from build123d import *

# Parameters (mm, degrees)
BOSS_EXTRUDE1_DEPTH = 5.4
SKETCH3_W           = 0.6
SKETCH3_H           = 0.5
BOSS_EXTRUDE3_DEPTH = 4.7
SKETCH4_W           = 2
SKETCH4_H           = 2
BOSS_EXTRUDE4_DEPTH = 2
SKETCH5_W           = 1.2
SKETCH5_H           = 2.4
CUT_EXTRUDE1_DEPTH  = 4.6


with BuildPart() as part:
    # Sketch1 → Boss-Extrude1 (new body)
    with BuildSketch(Plane(origin=(0, 0, 0), x_dir=(1, 0, 0), z_dir=(0, 1, 0))):
        with BuildLine():
            Line((-5.8, -2), (-0.3, -2))
            ThreePointArc((-0.3, -2), (0, -1.7), (0.3, -2))
            Line((0.3, -2), (5.8, -2))
            Line((5.8, -2), (5.8, 2))
            Line((5.8, 2), (0.3, 2))
            ThreePointArc((0.3, 2), (0, 1.7), (-0.3, 2))
            Line((-0.3, 2), (-5.8, 2))
            Line((-5.8, 2), (-5.8, -2))
        make_face()
    extrude(amount=BOSS_EXTRUDE1_DEPTH)

    # Sketch3 → Boss-Extrude3 (add)
    with BuildSketch(Plane.XZ):
        Rectangle(SKETCH3_W, SKETCH3_H)
        with Locations((2.5, 0)):
            Rectangle(SKETCH3_W, SKETCH3_H)
        with Locations((-2.5, 0)):
            Rectangle(SKETCH3_W, SKETCH3_H)
    extrude(amount=BOSS_EXTRUDE3_DEPTH)

    # Sketch4 → Boss-Extrude4 (add)
    with BuildSketch(Plane(origin=(0, 5.4, 0), x_dir=(1, 0, 0), z_dir=(0, 1, 0))):
        with Locations((-1.3, 0)):
            Rectangle(SKETCH4_W, SKETCH4_H)
    extrude(amount=BOSS_EXTRUDE4_DEPTH)

    # Sketch5 → Cut-Extrude1 (cut)
    with BuildSketch(Plane(origin=(0, 5.4, 0), x_dir=(1, 0, 0), z_dir=(0, 1, 0))):
        with Locations((5.8, 0)):
            Rectangle(SKETCH5_W, SKETCH5_H)
    cut_extrude1 = extrude(amount=-CUT_EXTRUDE1_DEPTH, mode=Mode.SUBTRACT)

    # Mirror1: Cut-Extrude1 across plane
    add(cut_extrude1.mirror(Plane(origin=(0, 0, 0), x_dir=(0, 0, 1), z_dir=(1, 0, 0))), mode=Mode.SUBTRACT)


solid = part.part
Geometry: final body of the model. Coordinates: model frame, mm. A direction names the side the tool comes from. Give positions to 0.01 mm unless a question says otherwise; leave off trailing zeros. Write each loop counter-clockwise with the first axis right and the second up, starting at its lowest first coordinate (ties: lowest second). Pieces come first, ordered by that corner, then holes. Notation, with made-up numbers: (11, 31.25) -> (47, 31.25) arc R20 ccw to (47, 62.25) -> close; hole circle Ø2 at (40, -34). An arc over 180 degrees is marked (long way). Answer as a JSON object with one key per item and string values.
1. Cut plane B-B on x = 2.5. Output: boundary loops of the cut face in (y, z).
Ans:
{"outline": "(-4.7, -0.25) -> (0, -0.25) -> (0, -2) -> (5.4, -2) -> (5.4, 2) -> (0, 2) -> (0, 0.25) -> (-4.7, 0.25) -> close"}
2. Cut plane D-D on z = -0.75. Output: boundary loops of the cut face in (x, y).
Ans:
{"outline": "(-5.8, 0) -> (5.8, 0) -> (5.8, 0.8) -> (5.2, 0.8) -> (5.2, 5.4) -> (-0.3, 5.4) -> (-0.3, 7.4) -> (-2.3, 7.4) -> (-2.3, 5.4) -> (-5.2, 5.4) -> (-5.2, 0.8) -> (-5.8, 0.8) -> close"}
3. Access query for faces 5 (the flat face through (-1, 6, -1)), 6 (the flat face through (-0.3, 6, 0)), 7 (the flat face through (-1, 6, 1)), 8 (the flat face through (3, 3, -2)). Directions: +Z, -Z, +X, -X, +Y, -Y. A direction counts if a zero-diameter tool reaches every point of the face in a straight line with its end or side. Return the directions, or none.
Ans:
{"face 5": "-Z, +X, -X, +Y", "face 6": "+Z, -Z, +X, +Y", "face 7": "+Z, +X, -X, +Y", "face 8": "-Z, +X, -X, +Y, -Y"}
4. Ray query, probe 1 along X at (y, z) = (-4, 0.2); probe 2 along Y at (x, z) = (0.75, 0.6); probe 3 along X at (y, z) = (2.5, -0.1). Return the intervals inside material, ascending. Write a range as from..to.
Ans:
{"probe 1": "x = -2.8..-2.2, -0.3..0.3, 2.2..2.8", "probe 2": "y = 0..5.4", "probe 3": "x = -5.2..5.2"}
5. Cut plane C-C on y = 2.5. Output: boundary loops of the cut face in (x, z).
Ans:
{"outline": "(-5.8, -2) -> (-0.3, -2) arc R0.3 cw to (0.3, -2) -> (5.8, -2) -> (5.8, -1.2) -> (5.2, -1.2) -> (5.2, 1.2) -> (5.8, 1.2) -> (5.8, 2) -> (0.3, 2) arc R0.3 cw to (-0.3, 2) -> (-5.8, 2) -> (-5.8, 1.2) -> (-5.2, 1.2) -> (-5.2, -1.2) -> (-5.8, -1.2) -> close"}
6. Cut plane A-A on y = -3. Output: boundary loops of the cut face in (x, z), and give its area (3 significant figures).
Ans:
{"outline": "(-2.8, -0.25) -> (-2.2, -0.25) -> (-2.2, 0.25) -> (-2.8, 0.25) -> close; (-0.3, -0.25) -> (0.3, -0.25) -> (0.3, 0.25) -> (-0.3, 0.25) -> close; (2.2, -0.25) -> (2.8, -0.25) -> (2.8, 0.25) -> (2.2, 0.25) -> close", "area": "0.900 mm^2"}
7. Contact query for flat-ended pins moving along their axis: pin 1 (1.6 mm diameter, centred on y = 7, z = 0, fed in from -X); pin 2 (1 mm diameter, centred on x = 3, z = 0, fed in from +Y); pin 3 (2 mm diameter, centred on x = 1.5, y = -2.5, fed in from +Z). Output: stop coordinate, or through.
Ans:
{"pin 1": "stops at x = -2.3", "pin 2": "stops at y = 5.4", "pin 3": "stops at z = 0.25"}
8. Mould query, pull axis Z, two halves, no side actions, for faces 1 (the flat face through (5.2, 3, 0)), 2 (the flat face through (-2.3, 6, 0)), 3 (the flat face through (-3, 3, 2)), 4 (the flat face through (-5.2, 3, 0)). Classes: pulls with the +Z half, pulls with the -Z half, needs draft (parallel to the pull), parting line crosses it, or undercut.
Ans:
{"face 1": "undercut", "face 2": "needs draft", "face 3": "pulls with the +Z half", "face 4": "undercut"}
